```python
from build123d import *

# Parameters (mm, degrees)
F0_W     = 0.5
F0_H     = 14.25
F0_H_2   = 12
F0_W_2   = 11.5
F0_H_3   = 0.5
F0_W_3   = 12
F1_DEPTH = 40
F2_DEPTH = 5
F3_SIZE  = 2
F5_DEPTH = 0.5


with BuildPart() as f1:
    # F0 (on Top) → F1 (new body)
    with BuildSketch(Plane.XY):
        Polygon((17.2627416998, 5.4343145751), (15, 3.1715728753), (15, -3.1715728753), (17.2627416998, -5.4343145751), (17.2627416998, -0.5656854249), (17.2627416998, 0.5656854249), align=None)
        Polygon((-15, 29.1715728753), (-15, 4.1715728753), (-12.1715728752, 7), (-12.1715728752, 0), (-12.1715728752, -7), (-15, -4.1715728753), (-15, -29.1715728753), (15, -29.1715728753), (15, -3.1715728753), (15, 3.1715728753), (15, 29.1715728753), align=None)
        Polygon((-10.4999961331, 14.999999851), (-10.4999961331, 26.999999851), (1.5000038669, 26.999999851), (2.0000038669, 26.999999851), (13.5000038669, 26.999999851), (13.5000038669, 14.999999851), (13.5000038669, 14.499999851), (13.5000038669, 0.249999851), (13.5000038669, -0.250000149), (13.5000038669, -14.500000149), (13.5000038669, -15.000000149), (13.5000038669, -27.000000149), (2.0000038669, -27.000000149), (1.5000038669, -27.000000149), (-10.4999961331, -27.000000149), (-10.4999961331, -15.000000149), (-10.4999961331, -14.500000149), (-10.4999961331, -0.250000149), (-10.4999961331, 0.249999851), (-10.4999961331, 14.499999851), align=None, mode=Mode.SUBTRACT)
        with Locations((1.7500038669, -7.375000149)):
            Rectangle(F0_W, F0_H)
        with Locations((1.7500038669, 20.999999851)):
            Rectangle(F0_W, F0_H_2)
        with Locations((7.7500038669, 14.749999851)):
            Rectangle(F0_W_2, F0_H_3)
        with Locations((-4.4999961331, -1.49e-07)):
            Rectangle(F0_W_3, F0_H_3)
        with Locations((7.7500038669, -1.49e-07)):
            Rectangle(F0_W_2, F0_H_3)
        with Locations((7.7500038669, -14.750000149)):
            Rectangle(F0_W_2, F0_H_3)
        with Locations((-4.4999961331, -14.750000149)):
            Rectangle(F0_W_3, F0_H_3)
        with Locations((-4.4999961331, 14.749999851)):
            Rectangle(F0_W_3, F0_H_3)
        with Locations((1.7500038669, 7.374999851)):
            Rectangle(F0_W, F0_H)
        with Locations((1.7500038669, -21.000000149)):
            Rectangle(F0_W, F0_H_2)
        with Locations((1.7500038669, -14.750000149)):
            Rectangle(F0_W, F0_H_3)
        with Locations((1.7500038669, -1.49e-07)):
            Rectangle(F0_W, F0_H_3)
        with Locations((1.7500038669, 14.749999851)):
            Rectangle(F0_W, F0_H_3)
    extrude(amount=F1_DEPTH)

    # F0 (on Top) → F2 (join)
    with BuildSketch(Plane.XY):
        Polygon((-15, 29.1715728753), (-15, 4.1715728753), (-12.1715728752, 7), (-12.1715728752, 0), (-12.1715728752, -7), (-15, -4.1715728753), (-15, -29.1715728753), (15, -29.1715728753), (15, -3.1715728753), (15, 3.1715728753), (15, 29.1715728753), align=None)
        Polygon((-10.4999961331, 14.999999851), (-10.4999961331, 26.999999851), (1.5000038669, 26.999999851), (2.0000038669, 26.999999851), (13.5000038669, 26.999999851), (13.5000038669, 14.999999851), (13.5000038669, 14.499999851), (13.5000038669, 0.249999851), (13.5000038669, -0.250000149), (13.5000038669, -14.500000149), (13.5000038669, -15.000000149), (13.5000038669, -27.000000149), (2.0000038669, -27.000000149), (1.5000038669, -27.000000149), (-10.4999961331, -27.000000149), (-10.4999961331, -15.000000149), (-10.4999961331, -14.500000149), (-10.4999961331, -0.250000149), (-10.4999961331, 0.249999851), (-10.4999961331, 14.499999851), align=None, mode=Mode.SUBTRACT)
        Polygon((-12.1715728752, 7), (-15, 4.1715728753), (-15, -4.1715728753), (-12.1715728752, -7), (-12.1715728752, 0), align=None)
        with Locations((1.7500038669, -21.000000149)):
            Rectangle(F0_W, F0_H_2)
        with Locations((7.7500038669, -21.000000149)):
            Rectangle(F0_W_2, F0_H_2)
        with Locations((-4.4999961331, -21.000000149)):
            Rectangle(F0_W_3, F0_H_2)
        with Locations((-4.4999961331, -14.750000149)):
            Rectangle(F0_W_3, F0_H_3)
        with Locations((1.7500038669, -14.750000149)):
            Rectangle(F0_W, F0_H_3)
        with Locations((1.7500038669, -7.375000149)):
            Rectangle(F0_W, F0_H)
        with Locations((-4.4999961331, -7.375000149)):
            Rectangle(F0_W_3, F0_H)
        with Locations((7.7500038669, -7.375000149)):
            Rectangle(F0_W_2, F0_H)
        with Locations((7.7500038669, 7.374999851)):
            Rectangle(F0_W_2, F0_H)
        with Locations((-4.4999961331, 7.374999851)):
            Rectangle(F0_W_3, F0_H)
        with Locations((1.7500038669, -1.49e-07)):
            Rectangle(F0_W, F0_H_3)
        with Locations((1.7500038669, 7.374999851)):
            Rectangle(F0_W, F0_H)
        with Locations((7.7500038669, 14.749999851)):
            Rectangle(F0_W_2, F0_H_3)
        with Locations((1.7500038669, 14.749999851)):
            Rectangle(F0_W, F0_H_3)
        with Locations((-4.4999961331, 14.749999851)):
            Rectangle(F0_W_3, F0_H_3)
        with Locations((-4.4999961331, 20.999999851)):
            Rectangle(F0_W_3, F0_H_2)
        with Locations((7.7500038669, 20.999999851)):
            Rectangle(F0_W_2, F0_H_2)
        with Locations((1.7500038669, 20.999999851)):
            Rectangle(F0_W, F0_H_2)
        with Locations((-4.4999961331, -1.49e-07)):
            Rectangle(F0_W_3, F0_H_3)
        with Locations((7.7500038669, -1.49e-07)):
            Rectangle(F0_W_2, F0_H_3)
        with Locations((7.7500038669, -14.750000149)):
            Rectangle(F0_W_2, F0_H_3)
    extrude(amount=-F2_DEPTH)

    # F3
    f3_edges = [f1.edges().sort_by_distance(p)[0] for p in [
        (0, -29.171573, -5),
        (0, 29.171573, -5),
        (0, -29.171573, 40),
        (0, 29.171573, 40),
    ]]
    chamfer(f3_edges, length=F3_SIZE)

    # F4 (on face) → F5 (cut)
    with BuildSketch(Plane(origin=(-12.1715728752, 0, 0), x_dir=(0, -1, 0), z_dir=(-1, 0, 0))):
        with BuildLine():
            Line((0.12, 10.25), (0.12, 10.5))
            ThreePointArc((0.12, 10.5), (-1.8790989856, 8.5600270426), (0, 6.5036032458))
            Line((0, 6.5036032458), (0, 6.7541191335))
            ThreePointArc((0, 6.7541191335), (-1.6289699135, 8.5600353381), (0.12, 10.25))
        make_face()
        with BuildLine():
            Line((0, 8.5), (0, 6.7541191335))
            ThreePointArc((0, 6.7541191335), (0.1250128042, 6.7500071795), (0.25, 6.7548352513))
            Line((0.25, 6.7548352513), (0.25, 8.25))
            Line((0.25, 8.25), (1.8520508076, 8.25))
            ThreePointArc((1.8520508076, 8.25), (1.865506934, 8.3746782406), (1.87, 8.5))
            Line((1.87, 8.5), (0, 8.5))
        make_face()
        with BuildLine():
            Line((0.25, 6.7548352513), (0.25, 6.5042294721))
            ThreePointArc((0.25, 6.5042294721), (1.5794519519, 7.1325205669), (2.12, 8.5))
            Line((2.12, 8.5), (1.87, 8.5))
            ThreePointArc((1.87, 8.5), (1.865506934, 8.3746782406), (1.8520508076, 8.25))
            ThreePointArc((1.8520508076, 8.25), (1.3140216535, 7.2206203491), (0.25, 6.7548352513))
        make_face()
        with BuildLine():
            Line((0, 6.7541191335), (0, 6.5036032458))
            ThreePointArc((0, 6.5036032458), (0.1250097944, 6.5000062745), (0.25, 6.5042294721))
            Line((0.25, 6.5042294721), (0.25, 6.7548352513))
            ThreePointArc((0.25, 6.7548352513), (0.1250128042, 6.7500071795), (0, 6.7541191335))
        make_face()
        with BuildLine():
            ThreePointArc((0.25, 6.5042294721), (0.1250097944, 6.5000062745), (0, 6.5036032458))
            Line((0, 6.5036032458), (0, 5))
            Line((0, 5), (0.25, 5))
            Line((0.25, 5), (0.25, 6.5042294721))
        make_face()
    extrude(amount=-F5_DEPTH, mode=Mode.SUBTRACT)


solid = f1.part
```
Verification items for the finished model (mm, model axes). Round coordinates to 2 decimals unless told otherwise and drop trailing zeros. Order: outer loops, then holes, each group sorted by start corner. A loop starts at its lowest first (then second) coordinate and runs counter-clockwise, first axis right, second up.
1) Depth check by flat-ended pin: pin 1 (3.5 mm diameter, centred on x = 7, y = 23.5, fed in from +Z); pin 2 (0.7 mm diameter, centred on y = -1, z = 7, fed in from -X); pin 3 (3 mm diameter, centred on y = 12, z = 20, fed in from +X). Enter the tip coordinate at first touch or a pass-through.
Geometry says:
pin 1: stops at z = 0
pin 2: stops at x = -12.17
pin 3: stops at x = 15
2) Material ranges on line 1 (Y direction, x = -7, z = 11.5); line 2 (X direction, y = 19.5, z = 23); line 3 (Z direction, x = -7, y = 9.5), recorded low to high.
Geometry says:
line 1: y = -29.17 to -27, -15 to -14.5, -0.25 to 0.25, 14.5 to 15, 27 to 29.17
line 2: x = -15 to -10.5, 1.5 to 2, 13.5 to 15
line 3: z = -5 to 0
3) Cross-section at B-B, the plane z = 1. Give the number of separate pieces and of enclosed holes in the cut face, plus the area to 3 significant figures.
Geometry says:
separate pieces: 1
enclosed holes: 8
area: 504 mm2
4) Cross-section at C-C, the plane y = -1. Record the cut outline in (x, z), plus the area to 3 significant figures.
Geometry says:
outline: (-15, -5) - (15, -5) - (15, 0) - (17.26, 0) - (17.26, 40) - (13.5, 40) - (13.5, 0) - (2, 0) - (2, 40) - (1.5, 40) - (1.5, 0) - (-10.5, 0) - (-10.5, 40) - (-12.17, 40) - (-12.17, 8.5) - (-11.67, 8.5) - (-11.67, 8.25) - (-12.17, 8.25) - (-12.17, 6.99) - (-11.67, 6.99) - (-11.67, 6.7) - (-12.17, 6.7) - (-12.17, 0) - (-15, 0) - close
area: 387 mm2
5) Draft check along Y on faces 1 (the cylindrical face through (-11.925, -1.326, 7.232)), 2 (the flat face through (0, 29.172, 18)). Enter one of: +Y half, -Y half, draft (parallel to the pull), parting line (faces both ways), or undercut.
Geometry says:
face 1: undercut
face 2: +Y half
6) Cross-section at A-A, the plane x = 9.5. Record the cut outline in (y, z).
Geometry says:
outline: (-29.17, -3) - (-27.17, -5) - (27.17, -5) - (29.17, -3) - (29.17, 38) - (27.17, 40) - (27, 40) - (27, 0) - (15, 0) - (15, 40) - (14.5, 40) - (14.5, 0) - (0.25, 0) - (0.25, 40) - (-0.25, 40) - (-0.25, 0) - (-14.5, 0) - (-14.5, 40) - (-15, 40) - (-15, 0) - (-27, 0) - (-27, 40) - (-27.17, 40) - (-29.17, 38) - close
